Geometry check sheet. Reference: the model listing, model coordinates, mm. A direction names the side the tool comes from. Coordinates: 2 decimals unless noted, no trailing zeros. Loops run counter-clockwise (first coordinate to the right, second up) from the corner with the lowest first, then second, coordinate; pieces in that order, holes last. Notation, with made-up numbers: (-31, 18.25) -> (-11, 18.25) arc R22 cw to (-11, 50.25) -> close; hole circle Ø11 at (-40, -34). An arc over 180 degrees is marked (long way). Answer as a JSON object with one key per item and string values.
from build123d import *

# Parameters (mm, degrees)
SKETCH_1_R               = 55
EXTRUDE_1_DEPTH          = 10
SKETCH_2_R               = 40
SKETCH_2_R_2             = 29
EXTRUDE_2_DEPTH          = 58.3
SKETCH_3_R               = 29.8
SKETCH_3_R_2             = 29
EXTRUDE_3_DEPTH          = 3
SKETCH_6_W               = 20
SKETCH_6_H               = 20
CUT_EXTRUDE_3_DEPTH      = 55.5
PATTERN_CIRCULAR_1_COUNT = 4
SKETCH_9_R               = 1.7
CUT_EXTRUDE_6_DEPTH      = 10
SKETCH_10_R              = 29
SKETCH_10_R_2            = 18
EXTRUDE_4_DEPTH          = 10
SKETCH_11_R              = 1.7
CUT_EXTRUDE_7_DEPTH      = 10
SKETCH_12_R              = 29
CUT_EXTRUDE_8_DEPTH      = 10
SKETCH_13_W              = 160.430825531
SKETCH_13_H              = 122.201891545
CUT_EXTRUDE_9_DEPTH      = 6
SKETCH_14_R              = 3.7
CUT_EXTRUDE_10_DEPTH     = 5.5
CUT_EXTRUDE_11_DEPTH     = 5.5
FILLET_1_R               = 5


with BuildPart() as part:
    # 草图1 → 凸台-拉伸1 (new body)
    with BuildSketch(Plane(origin=(0, 0, 0), x_dir=(1, 0, 0), z_dir=(0, 1, 0))):
        Circle(SKETCH_1_R)
    extrude(amount=EXTRUDE_1_DEPTH)

    # 草图2 → 凸台-拉伸2 (add)
    with BuildSketch(Plane(origin=(0, 10, 0), x_dir=(1, 0, 0), z_dir=(0, 1, 0))):
        Circle(SKETCH_2_R)
        Circle(SKETCH_2_R_2, mode=Mode.SUBTRACT)
    extrude(amount=EXTRUDE_2_DEPTH)

    # 草图3 → 凸台-拉伸3 (add)
    with BuildSketch(Plane(origin=(0, 68.3, 0), x_dir=(1, 0, 0), z_dir=(0, 1, 0))):
        Circle(SKETCH_3_R)
        Circle(SKETCH_3_R_2, mode=Mode.SUBTRACT)
    extrude(amount=EXTRUDE_3_DEPTH)

    # 草图6 → 切除-拉伸3 (cut, symmetric)
    with BuildSketch(Plane(origin=(0, 0, 0), x_dir=(0, 0, -1), z_dir=(1, 0, 0))):
        with Locations((0, 20)):
            Rectangle(SKETCH_6_W, SKETCH_6_H)
    cut_extrude_3 = extrude(amount=CUT_EXTRUDE_3_DEPTH, both=True, mode=Mode.SUBTRACT)

    # 阵列(圆周)1: 切除-拉伸3 ×4 about axis
    pattern_circular_1_axis = Axis((0, 68.3, 0), (0, -1, 0))
    for i in range(1, PATTERN_CIRCULAR_1_COUNT):
        add(cut_extrude_3.rotate(pattern_circular_1_axis, i * 360 / PATTERN_CIRCULAR_1_COUNT), mode=Mode.SUBTRACT)

    # 草图9 → 切除-拉伸6 (cut)
    with BuildSketch(Plane.XZ):
        with Locations((50, 0)):
            Circle(SKETCH_9_R)
        with Locations((35.355339059, -35.355339059)):
            Circle(SKETCH_9_R)
        with Locations((0, -50)):
            Circle(SKETCH_9_R)
        with Locations((-35.355339059, -35.355339059)):
            Circle(SKETCH_9_R)
        with Locations((-50, 0)):
            Circle(SKETCH_9_R)
        with Locations((-35.355339059, 35.355339059)):
            Circle(SKETCH_9_R)
        with Locations((0, 50)):
            Circle(SKETCH_9_R)
        with Locations((35.355339059, 35.355339059)):
            Circle(SKETCH_9_R)
    extrude(amount=-CUT_EXTRUDE_6_DEPTH, mode=Mode.SUBTRACT)

    # 草图10 → 凸台-拉伸4 (add)
    with BuildSketch(Plane(origin=(0, 68.3, 0), x_dir=(1, 0, 0), z_dir=(0, 1, 0))):
        Circle(SKETCH_10_R)
        Circle(SKETCH_10_R_2, mode=Mode.SUBTRACT)
    extrude(amount=-EXTRUDE_4_DEPTH)

    # 草图11 → 切除-拉伸7 (cut)
    with BuildSketch(Plane(origin=(0, 68.3, 0), x_dir=(1, 0, 0), z_dir=(0, 1, 0))):
        with Locations((0, -25)):
            Circle(SKETCH_11_R)
        with Locations((-21.650635095, -12.5)):
            Circle(SKETCH_11_R)
        with Locations((-21.650635095, 12.5)):
            Circle(SKETCH_11_R)
        with Locations((0, 25)):
            Circle(SKETCH_11_R)
        with Locations((21.650635095, 12.5)):
            Circle(SKETCH_11_R)
        with Locations((21.650635095, -12.5)):
            Circle(SKETCH_11_R)
    extrude(amount=-CUT_EXTRUDE_7_DEPTH, mode=Mode.SUBTRACT)

    # 草图12 → 切除-拉伸8 (cut)
    with BuildSketch(Plane(origin=(0, 10, 0), x_dir=(1, 0, 0), z_dir=(0, 1, 0))):
        Circle(SKETCH_12_R)
    extrude(amount=-CUT_EXTRUDE_8_DEPTH, mode=Mode.SUBTRACT)

    # 草图13 → 切除-拉伸9 (cut)
    with BuildSketch(Plane.XZ):
        with Locations((1.79708664, -1.633715128)):
            Rectangle(SKETCH_13_W, SKETCH_13_H)
    extrude(amount=-CUT_EXTRUDE_9_DEPTH, mode=Mode.SUBTRACT)

    # 草图14 → 切除-拉伸10 (cut)
    with BuildSketch(Plane(origin=(0, 68.3, 0), x_dir=(1, 0, 0), z_dir=(0, 1, 0))):
        with Locations((21.650635095, 12.5)):
            Circle(SKETCH_14_R)
        with Locations((21.650635095, -12.5)):
            Circle(SKETCH_14_R)
        with Locations((0, -25)):
            Circle(SKETCH_14_R)
        with Locations((-21.650635095, -12.5)):
            Circle(SKETCH_14_R)
        with Locations((-21.650635095, 12.5)):
            Circle(SKETCH_14_R)
        with Locations((0, 25)):
            Circle(SKETCH_14_R)
    extrude(amount=-CUT_EXTRUDE_10_DEPTH, mode=Mode.SUBTRACT)

    # 草图15 → 切除-拉伸11 (cut)
    with BuildSketch(Plane(origin=(0, 10, 0), x_dir=(1, 0, 0), z_dir=(0, 1, 0))):
        Polygon((10, 10), (59.580067328, 10), (59.580067328, -10), (10, -10), (10, -56.748157484), (-10, -56.748157484), (-10, -10), (-60.120716696, -10), (-60.120716696, 10), (-10, 10), (-10, 63.130274599), (10, 63.130274599), align=None)
    extrude(amount=-CUT_EXTRUDE_11_DEPTH, mode=Mode.SUBTRACT)

    # 圆角1
    fillet_1_edges = [part.edges().sort_by_distance(p)[0] for p in [
        (28.284271247, 10, -28.284271247),
        (-28.284271247, 10, 28.284271247),
        (-28.284271247, 10, -28.284271247),
        (28.284271247, 10, 28.284271247),
    ]]
    fillet(fillet_1_edges, radius=FILLET_1_R)


solid = part.part
1. Mould release check, pull along X, two halves, no side actions. Record for faces 1 (the face through (-27, 6, 27)), 2 (the face through (34.006, 7.972, 34.321)), 3 (the face through (38.153, 41.277, -12.015)): released by +X, released by -X, zero draft, split by the parting line, or undercut.
Evaluation:
{"face 1": "zero draft", "face 2": "undercut", "face 3": "split by the parting line"}
2. Section check B-B, the plane x = -47. Record the boundary of the cut face in (y, z), then the cut area to 3 significant figures.
Evaluation:
{"outline": "(6, -28.57) -> (10, -28.57) -> (10, -10) -> (6, -10) -> close; (6, 10) -> (10, 10) -> (10, 28.57) -> (6, 28.57) -> close", "area": "149 mm^2"}
3. Section check D-D, the plane z = 12.5. State how many separate pieces and enclosed holes the cut face has, then the cut area to 3 significant figures.
Evaluation:
{"separate pieces": "4", "enclosed holes": "0", "area": "1,770 mm^2"}
4. Section check C-C, the plane y = 42.5. Record the boundary of the cut face in (x, z).
Evaluation:
{"outline": "circle Ø80 at (0, 0); hole circle Ø58 at (0, 0)"}
5. Tool access check on faces 4 (the face through (-34, 15, -10)), 5 (the face through (-34, 10, 34)), 6 (the face through (34, 10, 32)), 7 (the face through (25.18, 65.59, 11.39)), 8 (the face through (0, 30, 34)). Record the directions out of +Z, -Z, +X, -X, +Y, -Y that give a thin tool (end or side, any length) a straight path to the whole face; none if there is none.
Evaluation:
{"face 4": "+X, -X, -Y", "face 5": "+Z, -X, +Y", "face 6": "+Z, +X, +Y", "face 7": "+Y", "face 8": "+Z, -Z, -Y"}
6. Depth check by flat-ended pin: P1, Ø4.5, axis at x = 0, z = -25, coming from the +Y side; P2, Ø12, axis at y = 17.5, z = -37, coming from the -X side; P3, Ø5, axis at y = 24.5, z = -13.5, coming from the +X side; P4, Ø3, axis at x = 35.36, z = 35.36, coming from the -Y side. Enter the tip coordinate at first touch or a pass-through.
Evaluation:
{"P1": "stops at y = 62.8", "P2": "stops at x = -25.28", "P3": "stops at x = 38.46", "P4": "passes through"}
7. Section check A-A, the plane z = -47. Record the boundary of the cut face in (x, y).
Evaluation:
{"outline": "(-28.57, 6) -> (-10, 6) -> (-10, 10) -> (-28.57, 10) -> close; (10, 6) -> (28.57, 6) -> (28.57, 10) -> (10, 10) -> close"}
8. Thickness scan on probe 1 along X at (y, z) = (59.7, 12.5); probe 2 along X at (y, z) = (67.15, -12.5); probe 3 along X at (y, z) = (62.25, 0). Record the ranges inside material, lowest first. Write a range as from..to.
Evaluation:
{"probe 1": "x = -38..-23.35, -19.95..-12.95, 12.95..19.95, 23.35..38", "probe 2": "x = -38..-25.35, -17.95..-12.95, 12.95..17.95, 25.35..38", "probe 3": "x = -40..-18, 18..40"}
